Work out the finished part from the listing and answer in its coordinate system (mm). A direction names the side the tool comes from. Round coordinates to 2 decimals unless told otherwise and drop trailing zeros. Write each loop counter-clockwise with the first axis right and the second up, starting at its lowest first coordinate (ties: lowest second). Pieces come first, ordered by that corner, then holes. Notation, with made-up numbers: M 43,32.25 L 92,32.25 A19 ccw 92,44.25 Z; hole C -9.75,66.5 d6. An arc over 180 degrees is marked long. Answer in a Markdown table with one row per item.
```python
from build123d import *

# Parameters (mm, degrees)
BOSS_EXTRUDE1_DEPTH = 2
SKETCH2_R           = 4.5
SKETCH2_R_2         = 1.5
CUT_EXTRUDE1_DEPTH  = 2


with BuildPart() as part:
    # Sketch1 → Boss-Extrude1 (new body)
    with BuildSketch(Plane.XY):
        with BuildLine():
            Line((-13.3, 4.371498599), (-13.3, 18.3))
            Line((-13.3, 18.3), (-13.3, 19.084050384))
            ThreePointArc((-13.3, 19.084050384), (-9.834750168, 21.225119977), (-7, 18.3))
            Line((-7, 18.3), (7, 18.3))
            ThreePointArc((7, 18.3), (9.834750168, 21.225119977), (13.3, 19.084050384))
            Line((13.3, 19.084050384), (13.3, 18.3))
            Line((13.3, 18.3), (13.3, 4.371498599))
            ThreePointArc((13.3, 4.371498599), (14, 0), (13.3, -4.371498599))
            Line((13.3, -4.371498599), (13.3, -18.3))
            Line((13.3, -18.3), (13.3, -19.084050384))
            ThreePointArc((13.3, -19.084050384), (9.834750168, -21.225119977), (7, -18.3))
            Line((7, -18.3), (-7, -18.3))
            ThreePointArc((-7, -18.3), (-9.834750168, -21.225119977), (-13.3, -19.084050384))
            Line((-13.3, -19.084050384), (-13.3, -18.3))
            Line((-13.3, -18.3), (-13.3, -4.371498599))
            ThreePointArc((-13.3, -4.371498599), (-14, 0), (-13.3, 4.371498599))
        make_face()
    extrude(amount=BOSS_EXTRUDE1_DEPTH)

    # Sketch2 → Cut-Extrude1 (cut)
    with BuildSketch(Plane.XY.offset(2)):
        Circle(SKETCH2_R)
        with Locations((-10, 16.25)):
            Circle(SKETCH2_R_2)
        with Locations((10, 16.25)):
            Circle(SKETCH2_R_2)
        with Locations((-10, -16.25)):
            Circle(SKETCH2_R_2)
        with Locations((10, -16.25)):
            Circle(SKETCH2_R_2)
        with BuildLine():
            Line((3.889087297, 6.01040764), (6.01040764, 8.131727984))
            ThreePointArc((6.01040764, 8.131727984), (8.131727984, 8.131727984), (8.131727984, 6.01040764))
            Line((8.131727984, 6.01040764), (6.01040764, 3.889087297))
            ThreePointArc((6.01040764, 3.889087297), (3.889087297, 3.889087297), (3.889087297, 6.01040764))
        make_face()
        with BuildLine():
            Line((6.01040764, -3.889087297), (8.131727984, -6.01040764))
            ThreePointArc((8.131727984, -6.01040764), (8.131727984, -8.131727984), (6.01040764, -8.131727984))
            Line((6.01040764, -8.131727984), (3.889087297, -6.01040764))
            ThreePointArc((3.889087297, -6.01040764), (3.889087297, -3.889087297), (6.01040764, -3.889087297))
        make_face()
        with BuildLine():
            Line((-3.889087297, -6.01040764), (-6.01040764, -8.131727984))
            ThreePointArc((-6.01040764, -8.131727984), (-8.131727984, -8.131727984), (-8.131727984, -6.01040764))
            Line((-8.131727984, -6.01040764), (-6.01040764, -3.889087297))
            ThreePointArc((-6.01040764, -3.889087297), (-3.889087297, -3.889087297), (-3.889087297, -6.01040764))
        make_face()
        with BuildLine():
            Line((-6.01040764, 3.889087297), (-8.131727984, 6.01040764))
            ThreePointArc((-8.131727984, 6.01040764), (-8.131727984, 8.131727984), (-6.01040764, 8.131727984))
            Line((-6.01040764, 8.131727984), (-3.889087297, 6.01040764))
            ThreePointArc((-3.889087297, 6.01040764), (-3.889087297, 3.889087297), (-6.01040764, 3.889087297))
        make_face()
    extrude(amount=-CUT_EXTRUDE1_DEPTH, mode=Mode.SUBTRACT)


solid = part.part
```
1. The part is cut by section A-A (x = 0). Determine the outline of the cut face in (y, z), plus the area to 3 significant figures.
Calculated:
| item | result |
|---|---|
| outline | M -18.3,0 L -4.5,0 L -4.5,2 L -18.3,2 Z; M 4.5,0 L 18.3,0 L 18.3,2 L 4.5,2 Z |
| area | 55.2 mm² |
2. Determine the mould class of faces 5 (the flat face through (-13.3, 12, 1)), 6 (the flat face through (-4.965, 7.086, 1.014)), 7 (the flat face through (13.3, -12, 1)) for opening direction X: released by +X, released by -X, zero draft, split by the parting line, or undercut.
Calculated:
| item | result |
|---|---|
| face 5 | released by -X |
| face 6 | undercut |
| face 7 | released by +X |
3. Consider line 1 along Y through (x, z) = (-10, 0.55); line 2 along X through (y, z) = (15.5, 1.7); line 3 along Y through (x, z) = (-7.5, 0.9). Determine where each line is inside the solid, lowest interval first. Write a range as from..to.
Calculated:
| item | result |
|---|---|
| line 1 | y = -21.24..-17.75, -14.75..14.75, 17.75..21.24 |
| line 2 | x = -13.3..-11.3, -8.7..8.7, 11.3..13.3 |
| line 3 | y = -19.75..-8.51, -5.38..5.38, 8.51..19.75 |
4. Given pin 1 (1 mm diameter, centred on y = -14.5, z = 1.5, fed in from -X); pin 2 (1 mm diameter, centred on x = 1.5, z = 1, fed in from -Y); pin 3 (1.8 mm diameter, centred on x = -10, y = -16.25, fed in from +Z); pin 4 (0.6 mm diameter, centred on x = -3, z = 1.5, fed in from +Y), each flat-ended and moving along its own axis, determine where each tip first touches the part or whether it passes through.
Calculated:
| item | result |
|---|---|
| pin 1 | stops at x = -13.3 |
| pin 2 | stops at y = -18.3 |
| pin 3 | passes through |
| pin 4 | stops at y = 18.3 |
5. The part is cut by section B-B (y = 16.25). Determine the outline of the cut face in (x, z), plus the area to 3 significant figures.
Calculated:
| item | result |
|---|---|
| outline | M -13.3,0 L -11.5,0 L -11.5,2 L -13.3,2 Z; M -8.5,0 L 8.5,0 L 8.5,2 L -8.5,2 Z; M 11.5,0 L 13.3,0 L 13.3,2 L 11.5,2 Z |
| area | 41.2 mm² |
6. A tool of negligible diameter and unlimited length cuts with its end or side. For faces 1 (the flat face through (-13.3, -12, 1)), 2 (the cylindrical face through (-9.896, 21.232, 0.986)), 3 (the flat face through (7.056, -4.935, 1.014)), 4 (the flat face through (0, -18.3, 1)), from which of +Z, -Z, +X, -X, +Y, -Y can it reach the whole face along a straight path? Write none if from no direction.
Calculated:
| item | result |
|---|---|
| face 1 | +Z, -Z, -X, -Y |
| face 2 | +Z, -Z, +Y |
| face 3 | +Z, -Z |
| face 4 | +Z, -Z, -Y |
7. The part is cut by section C-C (y = 0). Determine the outline of the cut face in (x, z).
Calculated:
| item | result |
|---|---|
| outline | M -14,0 L -4.5,0 L -4.5,2 L -14,2 Z; M 4.5,0 L 14,0 L 14,2 L 4.5,2 Z |
8. The part is cut by section D-D (x = 10). Determine the outline of the cut face in (y, z).
Calculated:
| item | result |
|---|---|
| outline | M -21.24,0 L -17.75,0 L -17.75,2 L -21.24,2 Z; M -14.75,0 L 14.75,0 L 14.75,2 L -14.75,2 Z; M 17.75,0 L 21.24,0 L 21.24,2 L 17.75,2 Z |
